from build123d import *

# Parameters (mm, degrees)
CROQUIS1_W              = 22
CROQUIS1_H              = 6.35
SALIENTE_EXTRUIR1_DEPTH = 2.8067
SALIENTE_EXTRUIR2_DEPTH = 1.07696
SALIENTE_EXTRUIR2_TAPER = 3
REDONDEO1_R             = 0.049609375
CORTAR_EXTRUIR1_DEPTH   = 13.798873245


with BuildPart() as part:
    # Croquis1 → Saliente-Extruir1 (new body)
    with BuildSketch(Plane(origin=(0, 0, 0), x_dir=(1, 0, 0), z_dir=(0, 1, 0))):
        Rectangle(CROQUIS1_W, CROQUIS1_H)
    extrude(amount=SALIENTE_EXTRUIR1_DEPTH)

    # Croquis2 → Saliente-Extruir2 (add)
    with BuildSketch(Plane.ZY.offset(11)):
        Polygon((-0.993589744, 2.063091923), (-1.25, 2.063091923), (-1.25, 0.748989359), (-0.993589744, 0.748989359), (-0.993589744, 1.293861154), (1.25, 1.293861154), (1.25, 1.518220128), (-0.993589744, 1.518220128), align=None)
    extrude(amount=SALIENTE_EXTRUIR2_DEPTH, taper=SALIENTE_EXTRUIR2_TAPER)

    # Chaflán1: read off the stored shape, not the designer's step
    # Chaflán1: loft between two sections, ruled curve by curve
    chafl_n1_from = [
        Edge.make_line((-12.07696, 2.007207586, -1.194115663), (-12.07696, 0.804873696, -1.194115663)),
        Edge.make_line((-12.07696, 0.804873696, -1.194115663), (-12.07696, 0.804873696, -1.049474081)),
        Edge.make_line((-12.07696, 2.007207586, -1.194115663), (-12.07696, 2.007207586, -1.049474081)),
        Edge.make_line((-12.07696, 0.804873696, -1.049474081), (-12.07696, 1.349745491, -1.049474081)),
        Edge.make_line((-12.07696, 2.007207586, -1.049474081), (-12.07696, 1.462335791, -1.049474081)),
        Edge.make_line((-12.07696, 1.349745491, -1.049474081), (-12.07696, 1.349745491, 1.194115663)),
        Edge.make_line((-12.07696, 1.462335791, -1.049474081), (-12.07696, 1.462335791, 1.194115663)),
        Edge.make_line((-12.07696, 1.349745491, 1.194115663), (-12.07696, 1.462335791, 1.194115663)),
    ]
    chafl_n1_to = [
        Edge.make_line((-11, 2.628990732, -1.815898809), (-11, 0.18309055, -1.815898809)),
        Edge.make_line((-11, 0.18309055, -1.815898809), (-11, 0.18309055, -0.427690935)),
        Edge.make_line((-11, 2.628990732, -1.815898809), (-11, 2.628990732, -0.427690935)),
        Edge.make_line((-11, 0.18309055, -0.427690935), (-11, 0.727962345, -0.427690935)),
        Edge.make_line((-11, 2.628990732, -0.427690935), (-11, 2.084118937, -0.427690935)),
        Edge.make_line((-11, 0.727962345, -0.427690935), (-11, 0.727962345, 1.815898809)),
        Edge.make_line((-11, 2.084118937, -0.427690935), (-11, 2.084118937, 1.815898809)),
        Edge.make_line((-11, 0.727962345, 1.815898809), (-11, 2.084118937, 1.815898809)),
    ]
    chafl_n1 = Solid(Shell([*[Face.make_surface_from_curves(chafl_n1_from[k], chafl_n1_to[k]) for k in range(8)], Face(Wire(chafl_n1_from)), Face(Wire(chafl_n1_to))]))
    add(chafl_n1)

    # Redondeo1
    redondeo1_edges = [part.edges().sort_by_distance(p)[0] for p in [
        (-11.53848, 0.493982123, -1.505007236),
        (-11.53848, 2.318099159, -1.505007236),
        (-11.53848, 0.493982123, -0.738582508),
        (-11.53848, 2.318099159, -0.738582508),
        (-11.53848, 1.038853918, -0.738582508),
        (-11.53848, 1.773227364, -0.738582508),
        (-11.53848, 1.038853918, 1.505007236),
        (-11.53848, 1.773227364, 1.505007236),
    ]]
    fillet(redondeo1_edges, radius=REDONDEO1_R)

    # Croquis5 → Cortar-Extruir1 (cut, through all)
    with BuildSketch(Plane.XZ):
        with BuildLine():
            Line((-12.07696, -1.194115663), (-12.07696, 1.194115663))
            ThreePointArc((-12.07696, 1.194115663), (-11.963672899, 0), (-12.07696, -1.194115663))
        make_face()
    extrude(amount=-CORTAR_EXTRUIR1_DEPTH, mode=Mode.SUBTRACT)


solid = part.part
Can you work these out from the model? Positions are in its coordinate system, mm. A direction names the side the tool comes from. Give positions to 0.01 mm unless a question says otherwise; leave off trailing zeros. Order: outer loops, then holes, each group sorted by start corner. A loop starts at its lowest first (then second) coordinate and runs counter-clockwise, first axis right, second up. Notation, with made-up numbers: (89.5, 88.5) - (95.5, 88.5) arc R12 cw to (95.5, 93.5) - close; hole circle Ø4 at (36.5, -34). An arc over 180 degrees is marked (long way). Write each question's results on one line, items separated by ' | '.
1) Suppose I cut it at A-A, the plane z = 2.5. Write out the boundary of the cut face in (x, y), then the cut area to 3 significant figures.
Final values:
outline: (-11, 0) - (11, 0) - (11, 2.81) - (-11, 2.81) - close | area: 61.7 mm^2
2) Please list where these lines run through material, in increasing order: line 1 along X through (y, z) = (1.95, 2.5); line 2 along X through (y, z) = (1.85, -1). Write a range as [from, to].
Final values:
line 1: x = [-11, 11] | line 2: x = [-11.99, 11]
3) On a 3-axis mill with a long thin cutter (end or side, diameter ignored), from which of +Z, -Z, +X, -X, +Y, -Y can I reach the whole of each face in a straight line? I mean faces 1 (the face through (-11, 2.3, 0)), 2 (the face through (0, 0, 0)). Say none if no direction works.
Final values:
face 1: -X | face 2: +Z, -Z, +X, -X, -Y
